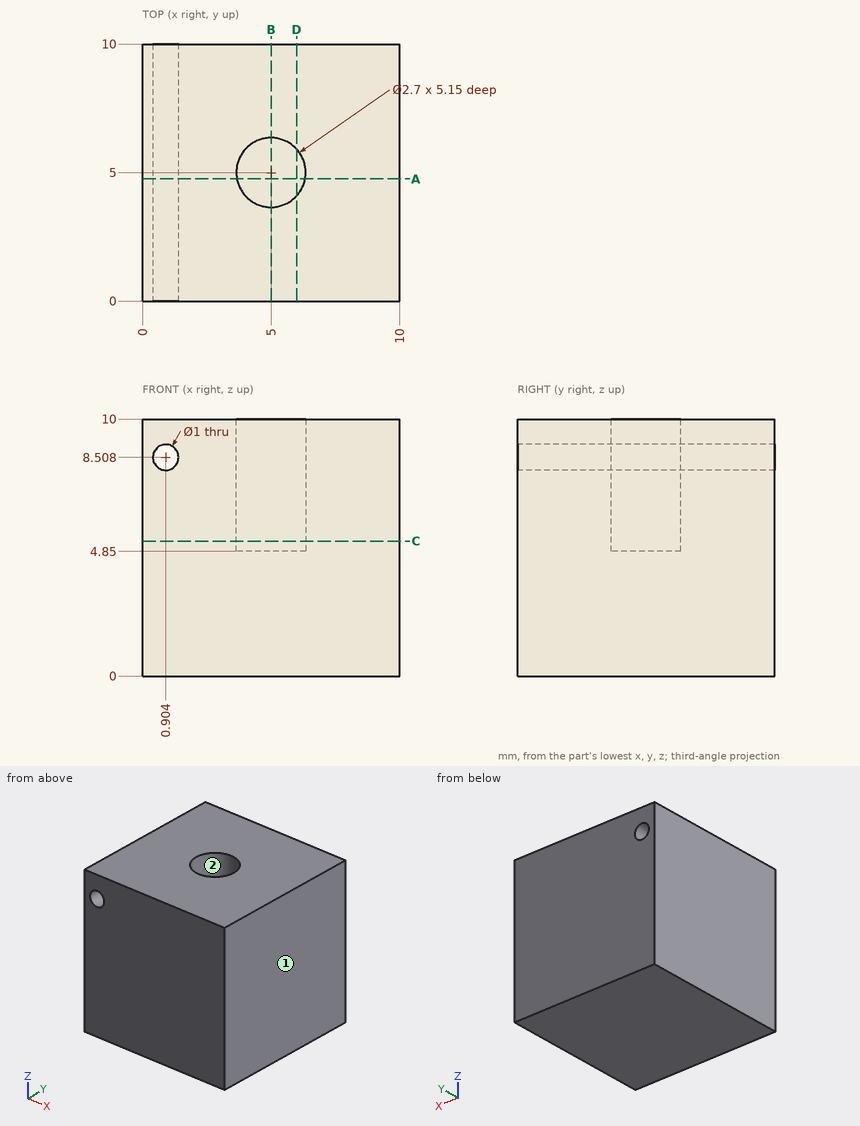
The drawing under review shows one solid part. Ordinate dimensions are in mm from its lowest x, y, z. A direction names the side the tool comes from. Round coordinates to 2 decimals unless told otherwise and drop trailing zeros. Write each loop counter-clockwise with the first axis right and the second up, starting at its lowest first coordinate (ties: lowest second). Pieces come first, ordered by that corner, then holes. Notation, with made-up numbers: (57.25, -5.5) -> (65.25, -5.5) arc R38 ccw to (65.25, 33.5) -> close; hole circle Ø8 at (46, 32). An arc over 180 degrees is marked (long way). Put each result on its own line as item: value.
Q1. Machinability: for the marked faces 1 and 2, which of the approach directions +Z, -Z, +X, -X, +Y, -Y give a long, thin tool a straight path to every point of the face, cutting with its end or side? Answer none if there is none.
Determined:
face 1: +Z, -Z, +X, +Y, -Y
face 2: +Z
Q2. Consider section B-B on x = 5. State the section outline as (y, z) points.
Determined:
outline: (0, 0) -> (10, 0) -> (10, 10) -> (6.35, 10) -> (6.35, 4.85) -> (3.65, 4.85) -> (3.65, 10) -> (0, 10) -> close
Q3. Consider section D-D on x = 6. State the section outline as (y, z) points.
Determined:
outline: (0, 0) -> (10, 0) -> (10, 10) -> (5.91, 10) -> (5.91, 4.85) -> (4.09, 4.85) -> (4.09, 10) -> (0, 10) -> close
Q4. Consider section C-C on z = 5.25. State the section outline as (x, y) points, and give its area (3 significant figures).
Determined:
outline: (0, 0) -> (10, 0) -> (10, 10) -> (0, 10) -> close; hole circle Ø2.7 at (5, 5)
area: 94.3 mm^2
Q5. Consider section A-A on y = 4.75. State the section outline as (x, z) points.
Determined:
outline: (0, 0) -> (10, 0) -> (10, 10) -> (6.33, 10) -> (6.33, 4.85) -> (3.67, 4.85) -> (3.67, 10) -> (0, 10) -> close; hole circle Ø1 at (0.9, 8.51)
Q6. To check wall thickness, follow L1, parallel to Y at x = 5, z = 7.7; L2, parallel to Y at x = 4, z = 6.75; L3, parallel to X at y = 5.5, z = 5. State the ranges of each line that lie inside material, in increasing order. Write a range as [from, to].
Determined:
L1: y = [0, 3.65], [6.35, 10]
L2: y = [0, 4.09], [5.91, 10]
L3: x = [0, 3.75], [6.25, 10]
